For this review, take the finished solid that the model builds, in its own axes (mm). A direction names the side the tool comes from. Coordinates: 2 decimals unless noted, no trailing zeros. Order: outer loops, then holes, each group sorted by start corner. A loop starts at its lowest first (then second) coordinate and runs counter-clockwise, first axis right, second up. Notation, with made-up numbers: (39, 83.5) -> (49, 83.5) arc R19 ccw to (49, 98.5) -> close; hole circle Ø3 at (2, 11). An arc over 180 degrees is marked (long way). Write item = value, one per line. Start each with the question number.
1) Consider section A-A on x = -2. Give the boundary of the cut face in (y, z), and give its area (3 significant figures).
2) Consider section C-C on z = 3.5. Give the boundary of the cut face in (x, y) (3 decimals), and give its area (3 significant figures).
3) Draft analysis for pull direction Z (two halves, no side actions). For faces 6 (the face through (0, 4, 7.298)), 7 (the face through (6.364, 4, -2)), 8 (the face through (3, 8.125, 3)), state which applies: +Z half, -Z half, draft (parallel to the pull), parting line (faces both ways), or undercut.
4) Consider section D-D on x = 2.5. Give the boundary of the cut face in (y, z) (3 decimals).
5) Wall thickness on probe 1 along Z at (x, y) = (-2, 8.5); probe 2 along Z at (x, y) = (1, 5.5); probe 3 along X at (y, z) = (7, -1.75): over which ranges is each line inside the solid? List them lowest first. Write a range as [from, to].
6) Machinability: for faces 1 (the face through (1, 2, 3.798)), 2 (the face through (4, 0, 0)), 3 (the face through (3, 0.875, 3)), 4 (the face through (3, 3.125, 3)), 5 (the face through (-6.436, 4, 6)), which of the approach directions +Z, -Z, +X, -X, +Y, -Y give a long, thin tool a straight path to every point of the face, cutting with its end or side? Answer none if there is none.
7) Consider section B-B on y = 2.5. Give the boundary of the cut face in (x, z).
8) Insertion check: pin 1 Ø1 at (x, z) = (2.5, 2.5) entering from -Y (3 decimals); pin 2 Ø2.5 at (y, z) = (3, -4.5) entering from -X; pin 3 Ø1.6 at (y, z) = (5.5, 2) entering from -X; pin 4 Ø1 at (x, z) = (1, 3) entering from +Y. Each pin has a flat end and moves straight along its axis. Give the tip position at first contact, or say it passes through.
Autodesk Inventor part; units mm, degrees
ref_plane "YZ Plane" through (0, 0, 0) normal (1, 0, 0) x (0, 1, 0)
ref_plane "XZ Plane" through (0, 0, 0) normal (0, 1, 0) x (-1, 0, 0)
ref_plane "XY Plane" through (0, 0, 0) normal (0, 0, 1) x (1, 0, 0)
sketch "Sketch1" plane through (0, 0, 0) normal (0, 1, 0) x (-1, 0, 0)
  line L0 (-3.364, -7.7022) -> (6.436, -7.7022)
  line L1 (6.436, -7.7022) -> (6.436, 4.2978)
  line L2 (6.436, 4.2978) -> (-3.364, 4.2978)
  line L3 (-3.364, 4.2978) -> (-3.364, -7.7022)
  line L4 (-3.364, -7.7022) -> (6.436, 4.2978) construction
  line L5 (6.436, -7.7022) -> (-3.364, 4.2978) construction
  line L6 (6.436, 4.2978) -> (6.436, 7.2978)
  line L7 (6.436, 7.2978) -> (-6.364, 7.2978)
  line L8 (-6.364, 7.2978) -> (-6.364, -10.7022)
  line L9 (-6.364, -10.7022) -> (6.436, -10.7022)
  line L10 (6.436, -10.7022) -> (6.436, -7.7022)
  point P0 (1.536, -1.7022)
  dimension "d27" = 12
  dimension "d28" = 9.8
  dimension "d29" = 3
  dimension "d30" = 3
extrude "Extrusion1" add sketch "Sketch1" along normal blind 9 contours L0 L10 L9 L8 L7 L6 L2 L3
sketch "Sketch2" plane through (0, 9, 0) normal (0, 1, 0) x (1, 0, 0)
  line L0 (3.364, -0.7978) -> (2.864, -0.7978)
  line L1 (2.864, -0.7978) -> (2.864, -2.2978)
  line L2 (-0.136, -4.2978) -> (-0.136, -3.7978)
  line L3 (-0.136, -4.2978) -> (0.364, -4.2978) construction
  line L4 (-0.136, -3.7978) -> (1.364, -3.7978)
  arc A0 (1.364, -3.7978) -> (2.864, -2.2978) centre (1.364, -2.2978) ccw
  line L5 (-0.136, -4.2978) -> (3.364, -4.2978)
  line L6 (3.364, -4.2978) -> (3.364, -0.7978)
  line L7 (3.364, 7.7022) -> (3.364, -4.2978)
  line L8 (3.364, -4.2978) -> (-6.436, -4.2978)
  point P0 (0, 0)
  point P1 (5, 6)
  point P2 (5, -6.1)
  dimension "d8" = 0.5
  dimension "d9" = 0.5
  dimension "d10" = 90
  dimension "d13" = 1.5
  dimension "d31" = 3.5
  dimension "d32" = 3.5
extrude "Extrusion2" add sketch "Sketch2" against normal up to surface (9 mm away)
sketch "Sketch3" plane through (-0.136, 9, 3.7978) normal (-1, 0, 0) x (0, 0, 1)
  line L0 (0.5, 0) -> (3.5, 0)
  line L1 (0.5, 0) -> (-3, 0)
  line L2 (-3, 0) -> (-3, -0.875)
  line L3 (-3, -0.875) -> (0.5, -0.875)
  line L4 (0.5, -0.875) -> (0.5, 0)
  line L5 (-3, 0) -> (-3, -9)
  line L6 (0.5, 0) -> (0.5, -9)
  line L7 (-3, -9) -> (-3, 0)
  line L8 (0.5, -9) -> (-3, -9)
  line L9 (-3, -9) -> (-3, -8.125)
  line L10 (-3, -8.125) -> (0.5, -8.125)
  line L11 (0.5, -8.125) -> (0.5, -9)
  line L12 (0.5, -5.875) -> (-3, -5.875)
  line L13 (-3, -5.875) -> (-3, -4.875)
  line L14 (-3, -4.875) -> (0.5, -4.875)
  line L15 (0.5, -4.875) -> (0.5, -5.875)
  point P0 (0.5, -8.125)
  point P1 (0.5, -4.875)
  dimension "d33" = 0.875
  dimension "d34" = 0.875
  dimension "d35" = 4
  dimension "d36" = 1
extrude "Extrusion3" cut sketch "Sketch3" against normal up to surface (3.5 mm away) contours L4 L3 L2 L1 | L6 L12 L5 L14 | L6 L8 L5 L10
properties part number "MotorMountTest"
Answer sheet:
q1.outline = (0, -10.7) -> (9, -10.7) -> (9, -7.7) -> (0, -7.7) -> close; (0, 4.3) -> (9, 4.3) -> (9, 7.3) -> (0, 7.3) -> close
q1.area = 54.0 mm2
q2.outline = (2.261, 0.875) -> (3.364, 0.875) -> (3.364, 0) -> (6.364, 0) -> (6.364, 9) -> (3.364, 9) -> (3.364, 8.125) -> (2.261, 8.125) -> (2.261, 4.125) -> (3.364, 4.125) -> (3.364, 3.125) -> (2.261, 3.125) -> close
q2.area = 33.9 mm2
q3.face_6 = +Z half
q3.face_7 = draft
q3.face_8 = undercut
q4.outline = (0, -10.702) -> (9, -10.702) -> (9, -7.702) -> (0, -7.702) -> close; (0, 4.298) -> (0.875, 4.298) -> (0.875, 3.277) -> (3.125, 3.277) -> (3.125, 4.298) -> (4.125, 4.298) -> (4.125, 3.277) -> (8.125, 3.277) -> (8.125, 4.298) -> (9, 4.298) -> (9, 7.298) -> (0, 7.298) -> close
q5.probe_1 = [-10.7, -7.7], [4.3, 7.3]
q5.probe_2 = [-10.7, -7.7], [3.8, 7.3]
q5.probe_3 = [3.36, 6.36]
q6.face_1 = -X, +Y, -Y
q6.face_2 = +Z, -Z, +X, -X, -Y
q6.face_3 = -X, -Y
q6.face_4 = -X
q6.face_5 = +Z, -Z, -X, +Y, -Y
q7.outline = (-6.44, -10.7) -> (6.36, -10.7) -> (6.36, 7.3) -> (-6.44, 7.3) -> (-6.44, 4.3) -> (-0.14, 4.3) -> (-0.14, 3.8) -> (1.36, 3.8) arc R1.5 cw to (2.86, 2.3) -> (2.86, 0.8) -> (3.36, 0.8) -> (3.36, -7.7) -> (-6.44, -7.7) -> close
q8.pin_1 = 0.875
q8.pin_2 = 3.36
q8.pin_3 = 2.78
q8.pin_4 = through
